Autodesk Inventor part; units mm, degrees
ref_plane "YZ Plane" through (0, 0, 0) normal (1, 0, 0) x (0, 1, 0)
ref_plane "XZ Plane" through (0, 0, 0) normal (0, 1, 0) x (-1, 0, 0)
ref_plane "XY Plane" through (0, 0, 0) normal (0, 0, 1) x (1, 0, 0)
sketch "Sketch1" plane through (0, 0, 0) normal (1, 0, 0) x (0, 1, 0)
  line L0 (-6.35, 6.35) -> (6.35, 6.35)
  line L1 (6.35, 6.35) -> (6.35, -6.35)
  line L2 (6.35, -6.35) -> (-6.35, -6.35)
  line L3 (-6.35, -6.35) -> (-6.35, 6.35)
  line L4 (-6.35, 6.35) -> (6.35, -6.35) construction
  line L5 (6.35, 6.35) -> (-6.35, -6.35) construction
  line L6 (-4.35, 4.35) -> (4.35, 4.35)
  line L7 (4.35, 4.35) -> (4.35, -4.35)
  line L8 (4.35, -4.35) -> (-4.35, -4.35)
  line L9 (-4.35, -4.35) -> (-4.35, 4.35)
  line L10 (-4.35, 4.35) -> (4.35, -4.35) construction
  line L11 (4.35, 4.35) -> (-4.35, -4.35) construction
  point P0 (0, 0)
  dimension "d0" = 12.7
  dimension "d1" = 12.7
  dimension "d13" = 2
  dimension "d14" = 2
extrude "Extrusion1" add sketch "Sketch1" along normal blind 170
sketch "Sketch2" plane through (0, 6.35, 6.35) normal (0, 1, 0) x (1, 0, 0)
  circle A0 centre (162, 5) radius 2.6
  line L0 (170, 12.7) -> (170, 0)
  circle A1 centre (142, 5) radius 2.6
  line L1 (0, 0) -> (170, 0)
  point P0 (0, 6.35)
  dimension "d8" = 5.2
  dimension "d9" = 8
  dimension "d10" = 5.2
  dimension "d11" = 20
  dimension "d12" = 5
extrude "Extrusion2" cut sketch "Sketch2" against normal blind 10
equation "\"d1\" = d0"
equation "\"d14\" = d13"
properties part number "arm"
Geometry check sheet. Reference: the model listing, model coordinates, mm. A direction names the side the tool comes from. Round coordinates to 2 decimals unless told otherwise and drop trailing zeros. Loops run counter-clockwise (first coordinate to the right, second up) from the corner with the lowest first, then second, coordinate; pieces in that order, holes last. Notation, with made-up numbers: (-27, -33.75) - (-17, -33.75) arc R6 ccw to (-17, -23.75) - close; hole circle Ø2 at (13.25, 16.25). An arc over 180 degrees is marked (long way). Write item = value, one per line. Start each with the question number.
1. Section check C-C on x = 92.5. Enter the section's corners in (y, z).
2. Depth check by flat-ended pin: pin 1 (3 mm diameter, centred on y = -4.5, z = 2, fed in from -X). Enter the tip coordinate at first touch or a pass-through.
3. Section check B-B on y = 0. Enter the section's corners in (x, z).
4. Set-up check for faces 1 (the face through (84, 6.35, 0)), 2 (the face through (144.4, 5.36, 2.35)), 3 (the face through (84, -4.35, 0)): record each of +Z, -Z, +X, -X, +Y, -Y from which the full face is reachable in a straight line by a thin tool's end or side.
5. Section check D-D on x = 142. Enter the section's corners in (y, z), then the cut area to 3 significant figures.
6. Section check A-A on z = 1.35. Enter the section's corners in (x, y), then the cut area to 3 significant figures.
7. Mould release check, pull along Y, two halves, no side actions. Record for faces 4 (the face through (84, 0, -4.35)), 5 (the face through (84, -6.35, 0)), 6 (the face through (0, 6, 0)): released by +Y, released by -Y, zero draft, split by the parting line, or undercut.
8. Thickness scan on line 1 (X direction, y = 5, z = 1.35); line 2 (Y direction, x = 122.5, z = 2.75); line 3 (Z direction, x = 142, y = 5.45). Record the ranges inside material, lowest first.
Working result:
q1.outline = (-6.35, -6.35) - (6.35, -6.35) - (6.35, 6.35) - (-6.35, 6.35) - close; hole (-4.35, -4.35) - (4.35, -4.35) - (4.35, 4.35) - (-4.35, 4.35) - close
q2.pin_1 = 0
q3.outline = (0, -6.35) - (170, -6.35) - (170, -4.35) - (0, -4.35) - close; (0, 4.35) - (170, 4.35) - (170, 6.35) - (0, 6.35) - close
q4.face_1 = +Z, -Z, +X, -X, +Y
q4.face_2 = +Y
q4.face_3 = +X, -X
q5.outline = (-6.35, -6.35) - (6.35, -6.35) - (6.35, -1.25) - (4.35, -1.25) - (4.35, -4.35) - (-4.35, -4.35) - (-4.35, 4.35) - (4.35, 4.35) - (4.35, 3.95) - (6.35, 3.95) - (6.35, 6.35) - (-6.35, 6.35) - close
q5.area = 75.2 mm^2
q6.outline = (0, -6.35) - (170, -6.35) - (170, -4.35) - (0, -4.35) - close; (0, 4.35) - (139.4, 4.35) - (139.4, 6.35) - (0, 6.35) - close; (144.6, 4.35) - (159.4, 4.35) - (159.4, 6.35) - (144.6, 6.35) - close; (164.6, 4.35) - (170, 4.35) - (170, 6.35) - (164.6, 6.35) - close
q6.area = 659 mm^2
q7.face_4 = undercut
q7.face_5 = released by -Y
q7.face_6 = zero draft
q8.line_1 = 0 to 139.4, 144.6 to 159.4, 164.6 to 170
q8.line_2 = -6.35 to -4.35, 4.35 to 6.35
q8.line_3 = -6.35 to -1.25, 3.95 to 6.35
